```python
from build123d import *

# Parameters (mm, degrees)
SKETCH1_W                     = 12
SKETCH1_H                     = 10
BOSS_EXTRUDE1_DEPTH           = 18
SKETCH5_R                     = 1.27
BOSS_EXTRUDE2_DEPTH           = 8
BOSS_EXTRUDE2_DRAFT           = 10
SKETCH5_2_R                   = 1.27
BOSS_EXTRUDE3_DEPTH           = 4
BOSS_EXTRUDE3_DRAFT           = 20
SKETCH5_4_R                   = 1.27
FILLET2_R                     = 15
SKETCH7_W                     = 12
SKETCH7_H                     = 11.5
BOSS_EXTRUDE4_DEPTH           = 4
SKETCH8_W                     = 12
SKETCH8_H                     = 3
BOSS_EXTRUDE5_DEPTH           = 6
SKETCH9_R                     = 1.375
CUT_EXTRUDE1_DEPTH            = 10
CUT_EXTRUDE2_REACH            = 39.682
CUT_EXTRUDE2_END_MAJOR_RADIUS = 4.5
CUT_EXTRUDE2_END_MINOR_RADIUS = 1.27
SKETCH10_R                    = 0.5
BOSS_EXTRUDE6_REACH           = 32.347
SKETCH11_W                    = 4
SKETCH11_H                    = 8.5
FILLET3_R                     = 1.5


with BuildPart() as part:
    # Sketch1 → Boss-Extrude1 (new body)
    with BuildSketch(Plane.XY):
        Rectangle(SKETCH1_W, SKETCH1_H)
    extrude(amount=BOSS_EXTRUDE1_DEPTH)

    # Sketch3 → Revolve1 (revolve)
    with BuildSketch(Plane(origin=(0, 0, 6.75), x_dir=(-1, 0, 0), z_dir=(0, 0, -1)), mode=Mode.PRIVATE) as revolve1_sk:
        with BuildLine():
            Line((-1.290509857, 5), (-2.27, 5))
            add(Edge.make_bspline(
                [(-5.5, 24.998503325), (-5.5, 24.807864043), (-5.459624999, 21.033247585), (-3.844625, 14.985265119), (-2.27, 8.510363101), (-2.27, 5)],
                knots=[0, 0, 0, 0, 0.025, 0.5, 1, 1, 1, 1], degree=3))
            ThreePointArc((-5.5, 24.998503325), (-4.990330513, 24.488833838), (-4.480661026, 24.998503325))
            Line((-4.480661026, 24.998503325), (-4.480661026, 23.998503325))
            add(Edge.make_bspline(
                [(-4.480661026, 23.998503325), (-4.46539815, 23.604834887), (-4.415661996, 22.80814634), (-4.253459846, 21.300457939), (-3.946721612, 19.489397713), (-3.463378936, 17.378771912), (-2.733557395, 14.546016044), (-1.989493801, 11.563267181), (-1.469127638, 8.442402152), (-1.323407915, 6.810453777), (-1.290509857, 6)],
                knots=[0.046251522, 0.046251522, 0.046251522, 0.046251522, 0.102999667, 0.159747812, 0.273244102, 0.386740392, 0.500236682, 0.727229262, 0.840725552, 0.954221841, 0.954221841, 0.954221841, 0.954221841], degree=3))
            Line((-1.290509857, 6), (-1.290509857, 5))
        make_face()
    revolve(revolve1_sk.sketch.rotate(Axis((0, 24.998503325, 6.75), (0, -1, 0)), 180), axis=Axis((0, 24.998503325, 6.75), (0, -1, 0)))


with BuildPart() as boss_extrude2_tool:
    # Sketch5 → Boss-Extrude2 (with draft: the straight prism first)
    with BuildSketch(Plane.ZY.offset(14)):
        with Locations((6.75, 0)):
            Circle(SKETCH5_R)
    extrude(amount=-BOSS_EXTRUDE2_DEPTH)
    # Boss-Extrude2: the draft: its side faces are tilted about the plane it starts from
    boss_extrude2_sides = [boss_extrude2_tool.faces().sort_by_distance(p)[0] for p in [
        (-10, 0, 5.48),
    ]]
    draft(boss_extrude2_sides, Plane.ZY.offset(14), BOSS_EXTRUDE2_DRAFT)


with BuildPart() as part_1:
    add(part.part)

    # Boss-Extrude2: add boss_extrude2_tool
    add(boss_extrude2_tool.part)


with BuildPart() as boss_extrude3_tool:
    # Sketch5<2> → Boss-Extrude3 (with draft: the straight prism first)
    with BuildSketch(Plane.ZY.offset(14)):
        with Locations((6.75, 0)):
            Circle(SKETCH5_2_R)
    extrude(amount=-BOSS_EXTRUDE3_DEPTH)
    # Boss-Extrude3: the draft: its side faces are tilted about the plane it starts from
    boss_extrude3_sides = [boss_extrude3_tool.faces().sort_by_distance(p)[0] for p in [
        (-12, 0, 5.48),
    ]]
    draft(boss_extrude3_sides, Plane.ZY.offset(14), BOSS_EXTRUDE3_DRAFT)


with BuildPart() as part_2:
    add(part_1.part)

    # Boss-Extrude3: add boss_extrude3_tool
    add(boss_extrude3_tool.part)

    # Cut-Sweep1: sweep along a path in Sketch6
    with BuildLine(Plane(origin=(0, 0, 6.75), x_dir=(-1, 0, 0), z_dir=(0, 0, -1))) as cut_sweep1_path:
        Line((14, 0), (4.5, 0))
        ThreePointArc((4.5, 0), (1.318019485, 1.318019485), (0, 4.5))
        Line((0, 4.5), (0, 5))
    # Sketch5<4> → Cut-Sweep1 (sweep, cut)
    with BuildSketch(Plane.ZY.offset(14)):
        with Locations((6.75, 0)):
            Circle(SKETCH5_4_R)
    sweep(path=cut_sweep1_path.line, mode=Mode.SUBTRACT)

    # Fillet1: read off the stored shape, not the designer's step
    # Fillet1 outline → Fillet1 (revolve, cut)
    with BuildSketch(Plane.XY.offset(6.75)):
        with BuildLine():
            ThreePointArc((1.27, 4.547586565), (1.275130096, 4.774025613), (1.290509857, 5))
            Line((1.290509857, 5), (1.27, 5))
            Line((1.27, 5), (1.27, 4.547586565))
        make_face()
    revolve(axis=Axis((0, 0, 6.75), (0, 1, 0)), mode=Mode.SUBTRACT)

    # Fillet2
    # the kernel refuses this fillet: 15 mm, written as the material it adds along each edge
    with BuildSketch(Plane(origin=(0, 5, 6.75), x_dir=(-1, 0, 0), z_dir=(0, 0, 1))) as fillet2_piece_1:
        with BuildLine():
            CenterArc((-13.709490143, -0.453110518), FILLET2_R, 0, 2.595022157)
            ThreePointArc((1.275127464, 0.226032446), (1.281538275, 0.112929088), (1.290509857, 0))
            Line((1.290509857, 0), (1.290509857, -0.453110518))
        make_face()
    revolve(axis=Axis((0, 5, 6.75), (0, -1, 0)), revolution_arc=180)
    with BuildSketch(Plane(origin=(0, 5, 6.75), x_dir=(1, 0, 0), z_dir=(0, 0, -1))) as fillet2_piece_2:
        with BuildLine():
            CenterArc((-13.709490143, -0.453110518), FILLET2_R, 360, 2.595022157)
            ThreePointArc((1.275127464, 0.226032446), (1.281538275, 0.112929088), (1.290509857, 0))
            Line((1.290509857, 0), (1.290509857, -0.453110518))
        make_face()
    revolve(axis=Axis((0, 5, 6.75), (0, -1, 0)), revolution_arc=180)

    # Sketch7 → Boss-Extrude4 (add)
    with BuildSketch(Plane.XY.offset(18)):
        with Locations((0, -10.75)):
            Rectangle(SKETCH7_W, SKETCH7_H)
    extrude(amount=-BOSS_EXTRUDE4_DEPTH)

    # Sketch8 → Boss-Extrude5 (add)
    with BuildSketch(Plane(origin=(0, 0, 14), x_dir=(-1, 0, 0), z_dir=(0, 0, -1))):
        with Locations((0, -15)):
            Rectangle(SKETCH8_W, SKETCH8_H)
    extrude(amount=BOSS_EXTRUDE5_DEPTH)

    # Sketch9 → Cut-Extrude1 (cut)
    with BuildSketch(Plane.XZ.offset(16.5)):
        with Locations(Location((0, 15.8, 0), (0, 0, 270))):
            Circle(SKETCH9_R)
    extrude(amount=-CUT_EXTRUDE1_DEPTH, mode=Mode.SUBTRACT)

    # Cut-Extrude2: up to this torus (the profile starts outside it)
    cut_extrude2_end = Plane(origin=(-4.5, 4.5, 6.75), z_dir=(0, 0, 1)) * Torus(CUT_EXTRUDE2_END_MAJOR_RADIUS, CUT_EXTRUDE2_END_MINOR_RADIUS, mode=Mode.PRIVATE)
    # Sketch10 → Cut-Extrude2 (cut, up to the surface)
    with BuildSketch(Plane.XZ.offset(5), mode=Mode.PRIVATE) as cut_extrude2_sk1:
        with Locations(Location((0, 6.75, 0), (0, 0, 270))):
            Circle(SKETCH10_R)
    cut_extrude2_tool1 = extrude(cut_extrude2_sk1.sketch, amount=-CUT_EXTRUDE2_REACH, mode=Mode.PRIVATE) - cut_extrude2_end
    add(cut_extrude2_tool1.solids().sort_by_distance((0, -5, 6.75))[0], mode=Mode.SUBTRACT)

    # Sketch11 → Boss-Extrude6 (add, up to next)
    with BuildSketch(Plane(origin=(0, 0, 8), x_dir=(-1, 0, 0), z_dir=(0, 0, -1)), mode=Mode.PRIVATE) as boss_extrude6_sk1:
        with Locations((4, -9.25)):
            Rectangle(SKETCH11_W, SKETCH11_H)
    boss_extrude6_tool1 = extrude(boss_extrude6_sk1.sketch, amount=-BOSS_EXTRUDE6_REACH, mode=Mode.PRIVATE) - part_2.part
    add(boss_extrude6_tool1.solids().sort_by_distance((-4, -9.25, 8))[0])

    # Fillet3
    fillet3_edges = [part_2.edges().sort_by_distance(p)[0] for p in [
        (-2, -13.5, 11),
        (-2, -5, 11),
    ]]
    fillet(fillet3_edges, radius=FILLET3_R)


solid = part_2.part
```
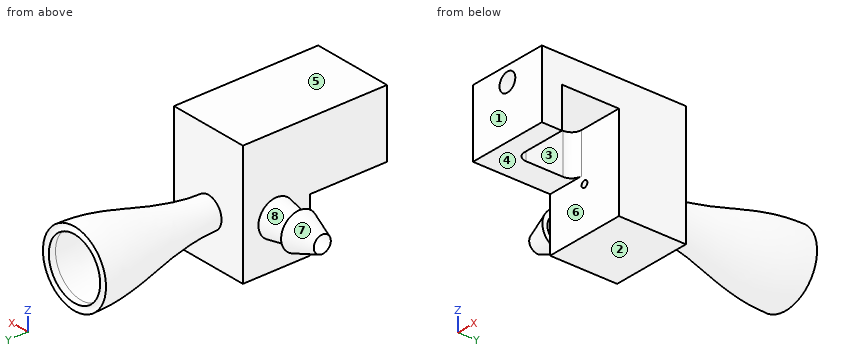
Can you work these out from the model? Positions are in its coordinate system, mm. Face numbers are marked on the shaded views. A direction names the side the tool comes from. Round coordinates to 2 decimals unless told otherwise and drop trailing zeros. Loops run counter-clockwise (first coordinate to the right, second up) from the corner with the lowest first, then second, coordinate; pieces in that order, holes last.
Item 1: If we mould it in two halves opening along Y, with no side actions, what happens to the marked faces 1, 2 and 3? For each: +Y half, -Y half, draft (parallel to the pull), parting line (faces both ways), or undercut.
Item 2: Will these pins go through, and if not, where does the flat tip stop? pin 1 Ø1.6 at (x, z) = (0, 15.8) entering from -Y; pin 2 Ø5.5 at (y, z) = (-4.5, 13.5) entering from -X; pin 3 Ø12 at (x, y) = (-2.5, 18) entering from +Z.
Item 3: Please list where these lines run through material, in increasing order: L1, parallel to Y at x = 5, z = 11.75; L2, parallel to X at y = -7, z = 13; L3, parallel to Y at x = 2.5, z = 15.
Item 4: Suppose I cut it at A-A, the plane z = 15.8. Write out the boundary of the cut face in (x, y) (3 decimals), then the cut area to 4 significant figures.
Item 5: Which directions (+Z, -Z, +X, -X, +Y, -Y) give clear straight access to the entire face, cutting with the end or side of a thin tool? Please do the marked faces 4, 5, 6, 7 and 8.
Item 6: Suppose I cut it at B-B, the plane y = -11.5. Write out the boundary of the cut face in (x, z) (3 decimals), then the cut area to 3 significant figures.
Reported:
1. face 1: -Y half
1. face 2: draft
1. face 3: undercut
2. pin 1: stops at y = -6.5
2. pin 2: stops at x = -6
2. pin 3: stops at z = 12.21
3. L1: y = -16.5 to -13.5, -5 to 5
3. L2: x = -6 to -2
3. L3: y = -16.5 to 5
4. outline: (-6, -16.5) - (-1.375, -16.5) - (-1.375, -6.5) - (1.375, -6.5) - (1.375, -16.5) - (6, -16.5) - (6, 5) - (-6, 5) - close
4. area: 230.5 mm2
5. face 4: -Z, +X, -X, -Y
5. face 5: +Z, +X, -X, +Y, -Y
5. face 6: -Z, +X
5. face 7: -X
5. face 8: none
6. outline: (-6, 8) - (-2, 8) - (-2, 14) - (6, 14) - (6, 18) - (-6, 18) - close; hole circle Ø2.75 at (0, 15.8)
6. area: 66.1 mm2
